Design review of the part built by this model. Coordinates are the model's own, in mm. Face numbers are marked on the shaded views. A direction names the side the tool comes from. Coordinates: 2 decimals unless noted, no trailing zeros. Loops run counter-clockwise (first coordinate to the right, second up) from the corner with the lowest first, then second, coordinate; pieces in that order, holes last. Notation, with made-up numbers: M -27,-3.5 L 21,-3.5 A27 ccw 21,13.5 Z; hole C 21.5,45.5 d6. An arc over 180 degrees is marked long. Answer as a JSON object with one key per item and string values. Group by question number.
1. Consider section A-A (z = -31.75). State the section outline as (x, y) points, then the cut area to 3 significant figures.
2. Consider section C-C (y = 10.25). State the section outline as (x, z) points, then the cut area to 3 significant figures.
3. Consider section D-D (x = 9.5). Count the separate pieces of the cut face and the enclosed holes in it, then the cut area to 3 significant figures.
4. To check wall thickness, follow probe 1 along X at (y, z) = (19.7, -31.75); probe 2 along Y at (x, z) = (7, -12); probe 3 along Z at (x, y) = (-9, 14.5). State the ranges of each line that lie inside material, in increasing order.
5. Insertion check: pin 1 (6 mm diameter, centred on x = 7, z = -20, fed in from -Y); pin 2 (6.5 mm diameter, centred on x = -8.73, y = 8.73, fed in from -Z). Each pin has a flat end and moves straight along its axis. Give the tip position at first contact, or say it passes through.
6. Machinability: for the marked faces 1 and 2, which of the approach directions +Z, -Z, +X, -X, +Y, -Y give a long, thin tool a straight path to every point of the face, cutting with its end or side? Answer none if there is none.
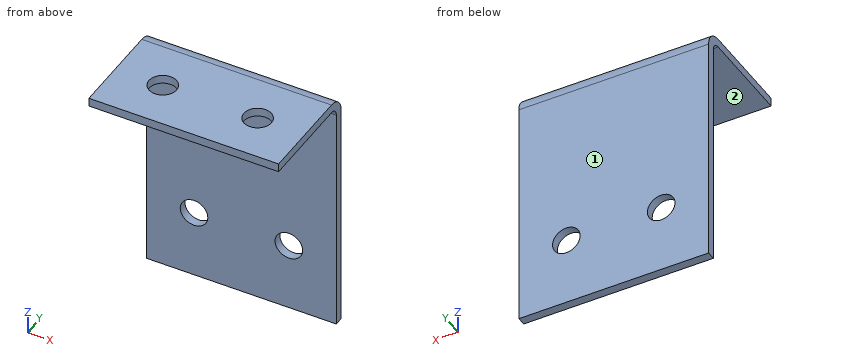
from build123d import *

# Parameters (mm, degrees)
BASE_FLANGE1_DEPTH = 17.4625
SKETCH6_R          = 2.54
CUT_EXTRUDE1_DEPTH = 2.54
SKETCH7_R          = 2.54
CUT_EXTRUDE2_DEPTH = 2.54


# Sheet-metal steps are written as plain solids
with BuildPart() as part:
    # Sketch1 → Base-Flange1 (new, symmetric)
    with BuildSketch(Plane(origin=(0, 0, 0), x_dir=(0, 0, -1), z_dir=(1, 0, 0))):
        with BuildLine():
            Line((0, 0), (0, 17.4625))
            ThreePointArc((0, 17.4625), (0.464967985, 18.585032015), (1.5875, 19.05))
            Line((1.5875, 19.05), (44.45, 19.05))
            Line((44.45, 19.05), (44.45, 20.6375))
            Line((44.45, 20.6375), (1.5875, 20.6375))
            ThreePointArc((1.5875, 20.6375), (-0.65756403, 19.70756403), (-1.5875, 17.4625))
            Line((-1.5875, 17.4625), (-1.5875, 0))
            Line((-1.5875, 0), (0, 0))
        make_face()
    extrude(amount=BASE_FLANGE1_DEPTH, both=True)

    # Sketch6 → Cut-Extrude1 (cut)
    with BuildSketch(Plane.XY.offset(1.5875)):
        with Locations((-8.73125, 8.73125)):
            Circle(SKETCH6_R)
        with Locations((8.73125, 8.73125)):
            Circle(SKETCH6_R)
    extrude(amount=-CUT_EXTRUDE1_DEPTH, mode=Mode.SUBTRACT)

    # Sketch7 → Cut-Extrude2 (cut)
    with BuildSketch(Plane(origin=(0, 20.6375, 0), x_dir=(1, 0, 0), z_dir=(0, 1, 0))):
        with Locations(Location((-8.73125, 31.75, 0), (0, 0, 270))):
            Circle(SKETCH7_R)
        with Locations(Location((8.73125, 31.75, 0), (0, 0, 270))):
            Circle(SKETCH7_R)
    extrude(amount=-CUT_EXTRUDE2_DEPTH, mode=Mode.SUBTRACT)


solid = part.part
Findings below:
{
 "1": {"outline": "M -17.46,19.05 L -11.27,19.05 L -11.27,20.64 L -17.46,20.64 Z; M -6.19,19.05 L 6.19,19.05 L 6.19,20.64 L -6.19,20.64 Z; M 11.27,19.05 L 17.46,19.05 L 17.46,20.64 L 11.27,20.64 Z", "area": "39.3 mm^2"},
 "2": {"outline": "M -17.46,0 L -10.77,0 L -10.77,1.59 L -17.46,1.59 Z; M -6.7,0 L 6.7,0 L 6.7,1.59 L -6.7,1.59 Z; M 10.77,0 L 17.46,0 L 17.46,1.59 L 10.77,1.59 Z", "area": "42.5 mm^2"},
 "3": {"separate pieces": "3", "enclosed holes": "0", "area": "86.3 mm^2"},
 "4": {"probe 1": "x = -17.46 to -11.27, -6.19 to 6.19, 11.27 to 17.46", "probe 2": "y = 19.05 to 20.64", "probe 3": "z = 0 to 1.59"},
 "5": {"pin 1": "stops at y = 19.05", "pin 2": "stops at z = 0"},
 "6": {"face 1": "+Z, -Z, +X, -X, +Y", "face 2": "-Z, +X, -X, -Y"}
}
